Design review of the part built by this model. Coordinates are the model's own, in mm. Round coordinates to 2 decimals unless told otherwise and drop trailing zeros. Write each loop counter-clockwise with the first axis right and the second up, starting at its lowest first coordinate (ties: lowest second). Pieces come first, ordered by that corner, then holes. Notation, with made-up numbers: M -14,8.25 L 14,8.25 A31 ccw 14,46.25 Z; hole C -10.75,-31 d10. An arc over 180 degrees is marked long. One line per question, with ' | ' between items. Start each with the question number.
Item 1: For L1, parallel to Y at x = -0.2, z = 1.5; L2, parallel to X at y = -144.5, z = -1.8; L3, parallel to Z at x = -4.5, y = -117.5, list the stretches that pass through material, from the lowest coordinate up.
Item 2: Add section B-B, the plane y = -220. State the section outline as (x, z) points.
Item 3: Insertion check: pin 1 Ø2.5 at (y, z) = (7, 2) entering from -X; pin 2 Ø0.9 at (y, z) = (7, 1) entering from +X; pin 3 Ø1 at (x, y) = (0.5, -141) entering from -Z. Each pin has a flat end and moves straight along its axis. Give the tip position at first contact, or say it passes through.
Item 4: Add section A-A, the plane z = -1.25. State the section outline as (x, y) points, and give its area (3 significant figures).
```python
from build123d import *

# Parameters (mm, degrees)
SKETCH2_W           = 6
SKETCH2_H           = 270
BOSS_EXTRUDE1_DEPTH = 3
BOSS_EXTRUDE2_DEPTH = 270
SKETCH5_W           = 3
SKETCH5_H           = 3
BOSS_EXTRUDE3_DEPTH = 10
SKETCH6_R           = 0.75
CUT_EXTRUDE1_DEPTH  = 40


with BuildPart() as part:
    # Sketch2 → Boss-Extrude1 (new body)
    with BuildSketch(Plane.XY):
        with Locations((-3, -135)):
            Rectangle(SKETCH2_W, SKETCH2_H)
    extrude(amount=BOSS_EXTRUDE1_DEPTH)

    # Sketch4 → Boss-Extrude2 (add)
    with BuildSketch(Plane(origin=(0, -270, 0), x_dir=(-1, 0, 0), z_dir=(0, -1, 0))):
        Polygon((0, 0), (-2.828427125, 2.828427125), (-2.828427125, -3), (0, -3), align=None)
        Polygon((8.828427125, -3), (6, -3), (6, 0), (8.828427125, 2.828427125), align=None)
    extrude(amount=-BOSS_EXTRUDE2_DEPTH)

    # Sketch5 → Boss-Extrude3 (add)
    with BuildSketch(Plane(origin=(0, 0, 0), x_dir=(1, 0, 0), z_dir=(0, 1, 0))):
        with Locations((-6.5, -1.5)):
            Rectangle(SKETCH5_W, SKETCH5_H)
        with Locations((0.5, -1.5)):
            Rectangle(SKETCH5_W, SKETCH5_H)
    extrude(amount=BOSS_EXTRUDE3_DEPTH)

    # Sketch6 → Cut-Extrude1 (cut)
    with BuildSketch(Plane(origin=(2, 0, 0), x_dir=(0, 0, -1), z_dir=(1, 0, 0))):
        with Locations((-1.5, 6)):
            Circle(SKETCH6_R)
    extrude(amount=-CUT_EXTRUDE1_DEPTH, mode=Mode.SUBTRACT)


solid = part.part
```
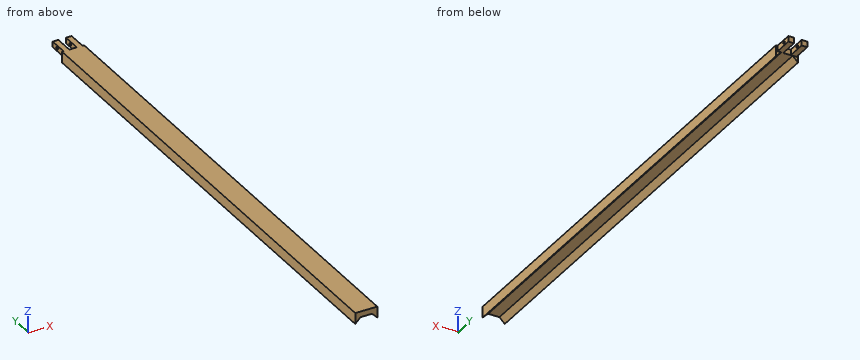
Computed values:
1) L1: y = -270 to 5.25, 6.75 to 10 | L2: x = -8.83 to -7.8, 1.8 to 2.83 | L3: z = 0 to 3
2) outline: M -8.83,-2.83 L -6,0 L 0,0 L 2.83,-2.83 L 2.83,3 L -8.83,3 Z
3) pin 1: stops at x = -8 | pin 2: stops at x = 2 | pin 3: stops at z = -1
4) outline: M -8.83,-270 L -7.25,-270 L -7.25,0 L -8.83,0 Z; M 1.25,-270 L 2.83,-270 L 2.83,0 L 1.25,0 Z | area: 852 mm^2
